Input: part model. Units: mm. Frame: model coordinates. Face numbers are marked on the shaded views. A direction names the side the tool comes from. Round coordinates to 2 decimals unless told otherwise and drop trailing zeros. Order: outer loops, then holes, each group sorted by start corner. A loop starts at its lowest first (then second) coordinate and runs counter-clockwise, first axis right, second up. Notation, with made-up numbers: (-35, 2.5) -> (-29, 2.5) arc R32 ccw to (-29, 35.5) -> close; hole circle Ø6 at (-33.5, 26.25). An arc over 180 degrees is marked (long way). Use a Markdown table: item, result.
from build123d import *

# Parameters (mm, degrees)
SKETCH1_R           = 2.95
BOSS_EXTRUDE1_DEPTH = 5.9
SKETCH2_R           = 17
CUT_EXTRUDE1_DEPTH  = 72.442524026
CUT_EXTRUDE2_DEPTH  = 72.442524026
FILLET1_R           = 10


with BuildPart() as part:
    # Sketch1 → Boss-Extrude1 (new body)
    with BuildSketch(Plane.XY):
        with BuildLine():
            Line((-15, -6.213203436), (-15, -24))
            Line((-15, -24), (15, -24))
            Line((15, -24), (15, 6.213203436))
            Line((15, 6.213203436), (-8.346024856, 29.559228292))
            ThreePointArc((-8.346024856, 29.559228292), (-44.194173824, 44.194173824), (-29.559228292, 8.346024856))
            Line((-29.559228292, 8.346024856), (-15, -6.213203436))
        make_face()
        Circle(SKETCH1_R, mode=Mode.SUBTRACT)
    extrude(amount=BOSS_EXTRUDE1_DEPTH)

    # Sketch2 → Cut-Extrude1 (cut, through all)
    with BuildSketch(Plane.XY.offset(5.9)):
        with Locations((-29.344931419, 29.344931419)):
            Circle(SKETCH2_R)
    extrude(amount=-CUT_EXTRUDE1_DEPTH, mode=Mode.SUBTRACT)

    # Sketch3 → Cut-Extrude2 (cut, through all)
    with BuildSketch(Plane.XY.offset(5.9)):
        Polygon((-9.15, -24), (-4.85, -24), (-4.85, -19), (-2.4, -19), (-2.4, -16), (-4.85, -16), (-4.85, -12), (-9.15, -12), (-9.15, -16), (-11.6, -16), (-11.6, -19), (-9.15, -19), align=None)
        Polygon((4.85, -16), (4.85, -12), (9.15, -12), (9.15, -16), (11.6, -16), (11.6, -19), (9.15, -19), (9.15, -24), (4.85, -24), (4.85, -19), (2.4, -19), (2.4, -16), align=None)
    extrude(amount=-CUT_EXTRUDE2_DEPTH, mode=Mode.SUBTRACT)

    # Fillet1
    fillet1_edges = [part.edges().sort_by_distance(p)[0] for p in [
        (-8.346024856, 29.559228292, 2.95),
        (15, 6.213203436, 2.95),
        (-15, -6.213203436, 2.95),
        (-29.559228292, 8.346024856, 2.95),
    ]]
    fillet(fillet1_edges, radius=FILLET1_R)


solid = part.part
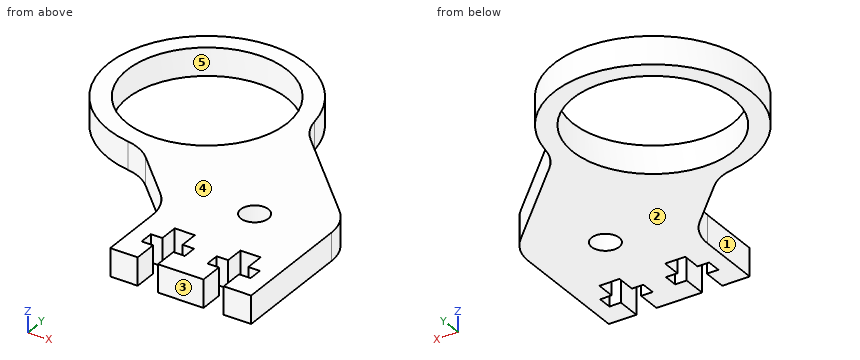
1) Cut plane B-B on x = -24. Return loops of the section in (y, z).
Results found:
| item | result |
|---|---|
| outline | (2.79, 0) -> (13.21, 0) -> (13.21, 5.9) -> (2.79, 5.9) -> close; (45.48, 0) -> (49.65, 0) -> (49.65, 5.9) -> (45.48, 5.9) -> close |
2) Cut plane D-D on y = 4.5. Return loops of the section in (x, z).
Results found:
| item | result |
|---|---|
| outline | (-25.71, 0) -> (14.7, 0) -> (14.7, 5.9) -> (-25.71, 5.9) -> close |
3) Line query: L1, parallel to X at y = -17, z = 4.05; L2, parallel to X at y = -19.5, z = 4.65; L3, parallel to X at y = 40, z = 1.1. Output: solid intervals per line, ascending. Write a range as [from, to].
Results found:
| item | result |
|---|---|
| L1 | x = [-15, -11.6], [-2.4, 2.4], [11.6, 15] |
| L2 | x = [-15, -9.15], [-4.85, 4.85], [9.15, 15] |
| L3 | x = [-47.44, -42.59], [-16.1, -11.25] |
4) Pull-direction query (Y, two-part tool) for the marked faces 3, 4 and 5; classes: +Y half, -Y half, draft (parallel to the pull), parting line (faces both ways), or undercut.
Results found:
| item | result |
|---|---|
| face 3 | -Y half |
| face 4 | draft |
| face 5 | undercut |
5) Cut plane C-C on z = 1.15. Count the separate pieces of the cut face and the enclosed holes in it, and give its area (3 significant figures).
Results found:
| item | result |
|---|---|
| separate pieces | 1 |
| enclosed holes | 2 |
| area | 1,710 mm² |
6) Pin query (flat end, axial travel): pin 1 Ø2.5 at (x, z) = (3.5, 2.5) entering from +Y; pin 2 Ø9.5 at (x, y) = (0, 0) entering from -Z; pin 3 Ø3.5 at (x, z) = (-7, 3) entering from -Y; pin 4 Ø20.5 at (x, y) = (-29.34, 29.34) entering from -Z (3 decimals). Return the tip coordinate at first contact, or that it passes through.
Results found:
| item | result |
|---|---|
| pin 1 | stops at y = 18.96 |
| pin 2 | stops at z = 0 |
| pin 3 | stops at y = -12 |
| pin 4 | passes through |
7) Set-up query: the marked faces 1 and 2. Return all of +Z, -Z, +X, -X, +Y, -Y with unobstructed straight access to the full face (end or side cutting, diameter ignored); none if empty.
Results found:
| item | result |
|---|---|
| face 1 | +Z, -Z, -X, -Y |
| face 2 | -Z, +X, -X, +Y, -Y |
8) Cut plane A-A on y = 34. Return loops of the section in (x, z), and give its area (3 significant figures).
Results found:
| item | result |
|---|---|
| outline | (-49.82, 0) -> (-45.7, 0) -> (-45.7, 5.9) -> (-49.82, 5.9) -> close; (-12.99, 0) -> (-8.87, 0) -> (-8.87, 5.9) -> (-12.99, 5.9) -> close |
| area | 48.7 mm² |
